Can you work these out from the drawing? Everything is in mm from the part's minimum corner. A direction names the side the tool comes from. Round coordinates to 2 decimals unless told otherwise and drop trailing zeros. Loops run counter-clockwise (first coordinate to the right, second up) from the corner with the lowest first, then second, coordinate; pieces in that order, holes last. Notation, with made-up numbers: (79.5, 1) -> (115.5, 1) arc R31 cw to (115.5, 29) -> close; hole circle Ø2 at (68, -11.5). An arc over 180 degrees is marked (long way). Answer as a JSON object with one key per item and string values.
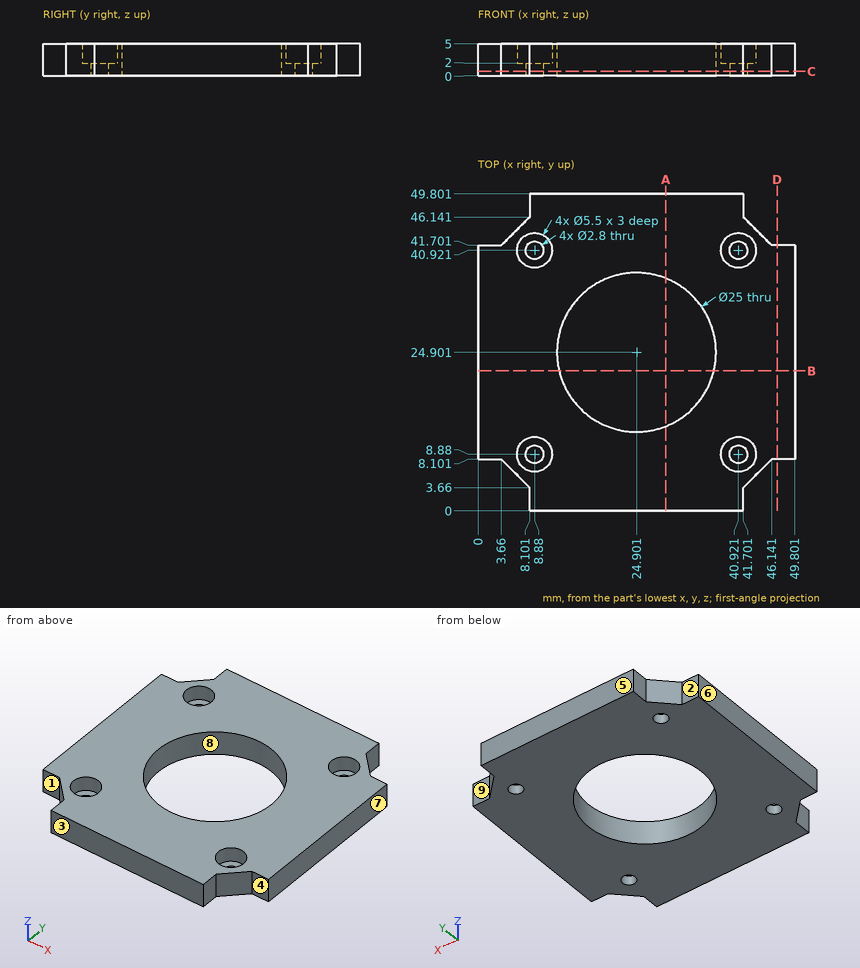
Q1. I want a section at B-B, the plane y = 22. Write out the boundary of the cut face in (x, z), then the cut area to 3 significant figures.
Determined:
{"outline": "(0, 0) -> (12.74, 0) -> (12.74, 5) -> (0, 5) -> close; (37.06, 0) -> (49.8, 0) -> (49.8, 5) -> (37.06, 5) -> close", "area": "127 mm²"}
Q2. I'm going to push flat-ended pins straight in: pin 1 (3.5 mm diameter, centred on x = 8.88, y = 40.92, fed in from -Z); pin 2 (1.8 mm diameter, centred on x = 1, z = 1.5, fed in from +Y); pin 3 (3 mm diameter, centred on y = 47, z = 3.5, fed in from +X); pin 4 (1.1 mm diameter, centred on y = 1.5, z = 2, fed in from +X). Where does each tip first touch, or does it pass through?
Determined:
{"pin 1": "z = 0", "pin 2": "y = 41.7", "pin 3": "x = 42.34", "pin 4": "x = 41.7"}
Q3. If I drill on L1, parallel to Y at x = 24.5, z = 3.45 (1 decimal); L2, parallel to X at y = 41.5, z = 0.35 (1 decimal); L3, parallel to X at y = 39.5, z = 4.15 (1 decimal), over which ranges is the centre line in solid material (lowest first)? Write a range as [from, to].
Determined:
{"L1": "[0, 12.4], [37.4, 49.8]", "L2": "[0, 7.6], [10.2, 39.6], [42.2, 49.8]", "L3": "[0, 6.5], [11.2, 38.6], [43.3, 49.8]"}
Q4. We'd pull the mould along X, two halves only. Please class the marked faces 6, 7, 8 and 9: pulls with the +X half, pulls with the -X half, needs draft (parallel to the pull), parting line crosses it, or undercut.
Determined:
{"face 6": "pulls with the -X half", "face 7": "pulls with the +X half", "face 8": "undercut", "face 9": "needs draft"}
Q5. I want a section at C-C, the plane z = 0.7. Write out the boundary of the cut face in (x, y), then the cut area to 3 significant figures.
Determined:
{"outline": "(0, 8.1) -> (3.66, 8.1) -> (8.1, 3.66) -> (8.1, 0) -> (41.7, 0) -> (41.7, 3.66) -> (46.14, 8.1) -> (49.8, 8.1) -> (49.8, 41.7) -> (46.14, 41.7) -> (41.7, 46.14) -> (41.7, 49.8) -> (8.1, 49.8) -> (8.1, 46.14) -> (3.66, 41.7) -> (0, 41.7) -> close; hole circle Ø2.8 at (8.88, 8.88); hole circle Ø2.8 at (8.88, 40.92); hole circle Ø25 at (24.9, 24.9); hole circle Ø2.8 at (40.92, 8.88); hole circle Ø2.8 at (40.92, 40.92)", "area": "1,740 mm²"}
Q6. I want a section at A-A, the plane x = 29.5. Write out the boundary of the cut face in (y, z).
Determined:
{"outline": "(0, 0) -> (13.28, 0) -> (13.28, 5) -> (0, 5) -> close; (36.52, 0) -> (49.8, 0) -> (49.8, 5) -> (36.52, 5) -> close"}
Q7. On a 3-axis mill with a long thin cutter (end or side, diameter ignored), from which of +Z, -Z, +X, -X, +Y, -Y can I reach the whole of each face in a straight line? I mean the marked faces 1, 2, 3, 4 and 5. Say none if no direction works.
Determined:
{"face 1": "+Z, -Z, -X, -Y", "face 2": "+Z, -Z, -X, +Y", "face 3": "+Z, -Z, +X, -X, -Y", "face 4": "+Z, -Z, +X, -Y", "face 5": "+Z, -Z, +X, -X, +Y"}
Q8. I want a section at D-D, the plane x = 47. Write out the boundary of the cut face in (y, z), then the cut area to 3 significant figures.
Determined:
{"outline": "(8.1, 0) -> (41.7, 0) -> (41.7, 5) -> (8.1, 5) -> close", "area": "168 mm²"}
